```python
from build123d import *

# Parameters (mm, degrees)
F1_DEPTH = 5
F3_DEPTH = 7


with BuildPart() as f1:
    # F0 (on Top) → F1 (new body)
    with BuildSketch(Plane.XY):
        Polygon((-25.4034118443, 44), (-50.8068236887, 0), (-25.4034118443, -44), (25.4034118443, -44), (50.8068236887, 0), (25.4034118443, 44), align=None)
        Polygon((-23.0940107676, -40), (-46.1880215352, 0), (-23.0940107676, 40), (23.0940107676, 40), (46.1880215352, 0), (23.0940107676, -40), align=None, mode=Mode.SUBTRACT)
        Polygon((-23.0940107676, 40), (-46.1880215352, 0), (-23.0940107676, -40), (23.0940107676, -40), (46.1880215352, 0), (23.0940107676, 40), align=None)
    extrude(amount=F1_DEPTH)

    # F2 (on face) → F3 (join)
    with BuildSketch(Plane.XY.offset(5)):
        Polygon((-25.4034118443, 44), (-50.8068236887, 0), (-25.4034118443, -44), (25.4034118443, -44), (50.8068236887, 0), (25.4034118443, 44), align=None)
        Polygon((-23.0940107676, -40), (-46.1880215352, 0), (-23.0940107676, 40), (23.0940107676, 40), (46.1880215352, 0), (23.0940107676, -40), align=None, mode=Mode.SUBTRACT)
    extrude(amount=F3_DEPTH)


solid = f1.part
```
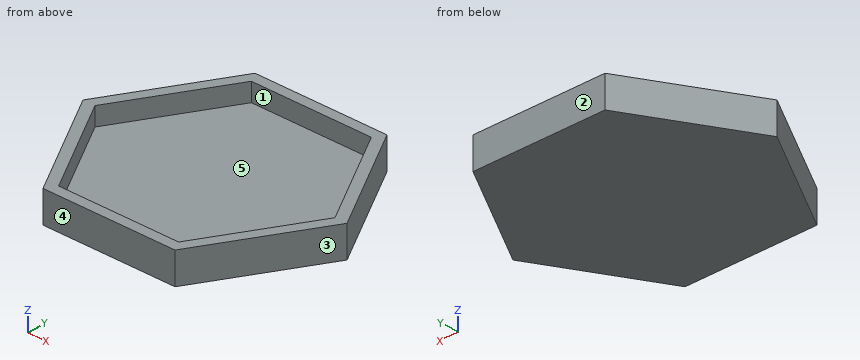
Can you work these out from the model? Positions are in its coordinate system, mm. Face numbers are marked on the shaded views. A direction names the side the tool comes from. Coordinates: 2 decimals unless noted, no trailing zeros. Loops run counter-clockwise (first coordinate to the right, second up) from the corner with the lowest first, then second, coordinate; pieces in that order, holes last. Notation, with made-up numbers: (82.5, -27) - (95.5, -27) arc R27 cw to (95.5, 0) - close; hole circle Ø8 at (36, -14.5). An arc over 180 degrees is marked (long way). Answer as CSV lines item,"result". Start each with the question number.
1) For pin 1 (8 mm diameter, centred on x = 29, y = -33.5, fed in from -Z), with a flat end and sliding along its axis, tell me the tip position at first contact or that it passes through.
2) I need wall thicknesses on line 1 (Y direction, x = 3.5, z = 5.5); line 2 (Z direction, x = 23, y = 0.5); line 3 (X direction, y = -10, z = 8.5). Which ranges of each line are inside material? Lowest first, please. Write a range as from..to.
3) Thinking about a two-plate mould opening in Y: for the marked faces 1, 2 and 3, which applies, pulls with the +Y half, pulls with the -Y half, needs draft (parallel to the pull), parting line crosses it, or undercut?
4) Suppose I cut it at C-C (y = 6). Please give me the cut outline in (x, z), plus the area to 3 significant figures.
5) Suppose I cut it at A-A (z = 8.5). Please give me the cut outline in (x, y).
6) Suppose I cut it at B-B (x = -40). Please give me the cut outline in (y, z).
7) Which directions (+Z, -Z, +X, -X, +Y, -Y) give clear straight access to the entire face, cutting with the end or side of a thin tool? Please do the marked faces 4 and 5.
8) Suppose I cut it at D-D (z = 1.5). Please give me the cut outline in (x, y).
Check result:
1,pin 1,"stops at z = 0"
2,line 1,"y = -44..-40, 40..44"
2,line 2,"z = 0..5"
2,line 3,"x = -45.03..-40.41, 40.41..45.03"
3,face 1,"undercut"
3,face 2,"pulls with the +Y half"
3,face 3,"pulls with the -Y half"
4,outline,"(-47.34, 0) - (47.34, 0) - (47.34, 12) - (42.72, 12) - (42.72, 5) - (-42.72, 5) - (-42.72, 12) - (-47.34, 12) - close"
4,area,"538 mm²"
5,outline,"(-50.81, 0) - (-25.4, -44) - (25.4, -44) - (50.81, 0) - (25.4, 44) - (-25.4, 44) - close; hole (-46.19, 0) - (-23.09, -40) - (23.09, -40) - (46.19, 0) - (23.09, 40) - (-23.09, 40) - close"
6,outline,"(-18.72, 0) - (18.72, 0) - (18.72, 12) - (10.72, 12) - (10.72, 5) - (-10.72, 5) - (-10.72, 12) - (-18.72, 12) - close"
7,face 4,"+Z, -Z, +X, -X, -Y"
7,face 5,"+Z"
8,outline,"(-50.81, 0) - (-25.4, -44) - (25.4, -44) - (50.81, 0) - (25.4, 44) - (-25.4, 44) - close"
